```python
from build123d import *

# Parameters (mm, degrees)
BOSS_EXTRUDE1_DEPTH = 28
CHAMFER1_START      = 34.535646335
CHAMFER1_OUTLINE_W  = 20
CHAMFER1_OUTLINE_H  = 22
CHAMFER1_DEPTH      = 9.464353665
CUT_EXTRUDE1_DEPTH  = 14


with BuildPart() as part:
    # Sketch1 → Boss-Extrude1 (new body)
    with BuildSketch(Plane(origin=(0, 0, 0), x_dir=(1, 0, 0), z_dir=(0, 1, 0))):
        Polygon((0, 0), (0, 7), (25, 7), (25, -21), (3.5, -21), (3.5, 0), align=None)
    extrude(amount=BOSS_EXTRUDE1_DEPTH)

    # Mirror1: part across plane


with BuildPart() as part_1:
    add(part.part)
    add(part.part.mirror(Plane(origin=(0, 28, 0), x_dir=(0, 0, 1), z_dir=(1, 0, 0))))

    # Chamfer1: read off the stored shape, not the designer's step
    # Chamfer1 outline → Chamfer1 (cut)
    with BuildSketch(Plane(origin=(0, 0, 0), x_dir=(0.8258790691262022, -0.39870024026782175, -0.39870024026782164), z_dir=(0.5638472871081651, 0.5839846902191711, 0.583984690219171)).offset(CHAMFER1_START)):
        with Locations((-2, 5)):
            Rectangle(CHAMFER1_OUTLINE_W, CHAMFER1_OUTLINE_H)
    extrude(amount=CHAMFER1_DEPTH, mode=Mode.SUBTRACT)

    # Sketch2 → Cut-Extrude1 (cut)
    with BuildSketch(Plane.ZY.offset(25)):
        Polygon((21, 28), (7, 28), (21, 14), align=None)
    extrude(amount=-CUT_EXTRUDE1_DEPTH, mode=Mode.SUBTRACT)


solid = part_1.part
```
Geometry check sheet. Reference: the model listing, model coordinates, mm. A direction names the side the tool comes from. Round coordinates to 2 decimals unless told otherwise and drop trailing zeros. Write each loop counter-clockwise with the first axis right and the second up, starting at its lowest first coordinate (ties: lowest second). Pieces come first, ordered by that corner, then holes. Notation, with made-up numbers: (77, 31.5) -> (81, 31.5) arc R19 cw to (81, 42.5) -> close; hole circle Ø10 at (59.5, 89.5). An arc over 180 degrees is marked (long way). Put each result on its own line as item: value.
1) Release check for a two-part mould opening along X. For faces 4 (the face through (19.26, 23.87, 16.67)), 5 (the face through (-3.5, 14, 11)), 6 (the face through (-12, 11, 21)) record: pulls with the +X half, pulls with the -X half, needs draft (parallel to the pull), parting line crosses it, or undercut.
Recorded:
face 4: pulls with the +X half
face 5: undercut
face 6: needs draft
2) Thickness scan on probe 1 along X at (y, z) = (7.5, 8.5); probe 2 along X at (y, z) = (18, 19.75); probe 3 along Z at (x, y) = (18, 24). Record the ranges inside material, lowest first. Write a range as from..to.
Recorded:
probe 1: x = -25..-3.5, 3.5..25
probe 2: x = -11..-3.5, 3.5..22.15
probe 3: z = -7..17.76
3) Cross-section at B-B, the plane y = 7. Enter the section's corners in (x, z), plus the area to 3 significant figures.
Recorded:
outline: (-25, -7) -> (25, -7) -> (25, 21) -> (3.5, 21) -> (3.5, 0) -> (-3.5, 0) -> (-3.5, 21) -> (-25, 21) -> close
area: 1,250 mm2
4) Cross-section at A-A, the plane z = 5.25. Enter the section's corners in (x, y).
Recorded:
outline: (-25, 0) -> (-3.5, 0) -> (-3.5, 28) -> (-25, 28) -> close; (3.5, 0) -> (25, 0) -> (25, 28) -> (3.5, 28) -> close
5) Depth check by flat-ended pin: P1, Ø8, axis at x = 18.5, z = 16, coming from the +Y side; P2, Ø2, axis at x = 0.5, y = 13, coming from the +Z side. Enter the tip coordinate at first touch or a pass-through.
Recorded:
P1: stops at y = 28
P2: stops at z = 0
6) Cross-section at D-D, the plane z = 15.25. Enter the section's corners in (x, y), plus the area to 3 significant figures.
Recorded:
outline: (-25, 0) -> (-3.5, 0) -> (-3.5, 28) -> (-11, 28) -> (-11, 19.75) -> (-25, 19.75) -> close; (3.5, 0) -> (25, 0) -> (25, 19.75) -> (16.46, 28) -> (3.5, 28) -> close
area: 1,050 mm2
7) Cross-section at C-C, the plane x = -17. Enter the section's corners in (y, z), plus the area to 3 significant figures.
Recorded:
outline: (0, -7) -> (28, -7) -> (28, 7) -> (14, 21) -> (0, 21) -> close
area: 686 mm2
8) Access from +Z, -Z, +X, -X, +Y, -Y to the whole of each face (thin tool, end or side, straight path). Record for faces 1 (the face through (-18, 21, 14)), 2 (the face through (25, 14, 7)), 3 (the face through (0, 14, 0)).
Recorded:
face 1: +Z, -X, +Y
face 2: +Z, -Z, +X, +Y, -Y
face 3: +Z, +Y, -Y
